Verification items for the finished model (mm, model axes). A direction names the side the tool comes from. Round coordinates to 2 decimals unless told otherwise and drop trailing zeros. Order: outer loops, then holes, each group sorted by start corner. A loop starts at its lowest first (then second) coordinate and runs counter-clockwise, first axis right, second up. Notation, with made-up numbers: (15, 15.25) -> (66, 15.25) arc R22 cw to (66, 24.25) -> close; hole circle Ø4 at (-31.75, -2.5). An arc over 180 degrees is marked (long way). Return JSON: item names as keys, results as strings. Group by question number.
1) Scan lines: L1, parallel to Z at x = 0, y = -3.5; L2, parallel to Z at x = 0, y = 2.65; L3, parallel to Y at x = 1.75, z = 3. Record each from-to range of solid material in increasing order.
2) Tool access check on faces 1 (the flat face through (-2, 5, -5)), 2 (the cylindrical face through (1.08, 2.46, 4.88)). Record the directions out of +Z, -Z, +X, -X, +Y, -Y that give a thin tool (end or side, any length) a straight path to the whole face; none if there is none.
3) Draft check along X on faces 3 (the cylindrical face through (5.158, -2.888, -3.955)), 4 (the cylindrical face through (2.579, -5.423, -1.978)), 5 (the flat face through (2, -11, 3)). Enter one of: pulls with the +X half, pulls with the -X half, needs draft (parallel to the pull), parting line crosses it, or undercut.
4) Section check A-A on x = 0. Enter the section's corners in (y, z).
5) Section check D-D on x = -3.5. Enter the section's corners in (y, z).
6) Section check B-B on z = 0. Enter the section's corners in (x, y).
7) Depth check by flat-ended pin: pin 1 (2 mm diameter, centred on x = 3.5, y = -6.5, fed in from +Z); pin 2 (3 mm diameter, centred on x = -2, z = 1.5, fed in from +Y); pin 3 (3 mm diameter, centred on x = -4.5, y = -0.5, fed in from +Z). Enter the tip coordinate at first touch or a pass-through.
8) Section check C-C on y = 3.75. Enter the section's corners in (x, z).
Autodesk Inventor part; units mm, degrees
ref_plane "YZ Plane" through (0, 0, 0) normal (1, 0, 0) x (0, 1, 0)
ref_plane "XZ Plane" through (0, 0, 0) normal (0, 1, 0) x (-1, 0, 0)
ref_plane "XY Plane" through (0, 0, 0) normal (0, 0, 1) x (1, 0, 0)
sketch "Sketch1" plane through (0, 0, 0) normal (0, 1, 0) x (-1, 0, 0)
  circle A0 centre (0, 0) radius 5
  circle A1 centre (0, 0) radius 6.5
  circle A2 centre (0, 0) radius 3.25
  dimension "d0" = 10
  dimension "d1" = 13
  dimension "d4" = 6.5
extrude "Extrusion5" add sketch "Sketch1" along normal blind 5 contours A1
extrude "Extrusion6" add sketch "Sketch1" against normal blind 11 contours A0 | A1
properties part number "clip_holder_ring"
Check result:
{
 "1": {"L1": "-6.5 to -3.25, 3.25 to 6.5", "L2": "-6.5 to -5, 5 to 6.5", "L3": "-11 to 0"},
 "2": {"face 1": "+Z, -Z, +X, -X, +Y", "face 2": "+Y"},
 "3": {"face 3": "parting line crosses it", "face 4": "undercut", "face 5": "needs draft"},
 "4": {"outline": "(-11, -6.5) -> (5, -6.5) -> (5, -5) -> (0, -5) -> (0, -3.25) -> (-11, -3.25) -> close; (-11, 3.25) -> (0, 3.25) -> (0, 5) -> (5, 5) -> (5, 6.5) -> (-11, 6.5) -> close"},
 "5": {"outline": "(-11, -5.48) -> (5, -5.48) -> (5, -3.57) -> (0, -3.57) -> (0, 3.57) -> (5, 3.57) -> (5, 5.48) -> (-11, 5.48) -> close"},
 "6": {"outline": "(-6.5, -11) -> (-3.25, -11) -> (-3.25, 0) -> (-5, 0) -> (-5, 5) -> (-6.5, 5) -> close; (3.25, -11) -> (6.5, -11) -> (6.5, 5) -> (5, 5) -> (5, 0) -> (3.25, 0) -> close"},
 "7": {"pin 1": "z = 6", "pin 2": "y = 0", "pin 3": "z = 5.77"},
 "8": {"outline": "circle Ø13 at (0, 0); hole circle Ø10 at (0, 0)"}
}
